For this review, take the finished solid that the model builds, in its own axes (mm). Round coordinates to 2 decimals unless told otherwise and drop trailing zeros. Write each loop counter-clockwise with the first axis right and the second up, starting at its lowest first coordinate (ties: lowest second). Pieces come first, ordered by that corner, then holes. Notation, with made-up numbers: (2, -25) -> (30, -25) arc R21 cw to (30, -6) -> close; hole circle Ø5 at (22, 34). An arc over 180 degrees is marked (long way). Answer in a Markdown table with one row per item. Add a question column.
```python
from build123d import *

# Parameters (mm, degrees)
SKETCH_1_W          = 17
SKETCH_1_H          = 14
SKETCH_1_R          = 1.1
EXTRUDE_1_DEPTH     = 3
EXTRUDE_3_DEPTH     = 3
SKETCH_3_R          = 1
CUT_EXTRUDE_1_DEPTH = 27.518861212
SKETCH_4_W          = 10
SKETCH_4_H          = 7
SKETCH_4_W_2        = 6
SKETCH_4_H_2        = 2
EXTRUDE_4_DEPTH     = 3
SKETCH_7_R          = 1
CUT_EXTRUDE_4_DEPTH = 27.518861212
FILLET_1_R          = 10
FILLET_2_R          = 2
CUT_EXTRUDE_5_DEPTH = 27.518861212


with BuildPart() as part:
    # 草图1 → 凸台-拉伸1 (new body)
    with BuildSketch(Plane(origin=(0, 0, 0), x_dir=(1, 0, 0), z_dir=(0, 1, 0))):
        Rectangle(SKETCH_1_W, SKETCH_1_H)
        with Locations(Location((-6, 4, 0), (0, 0, 270))):
            Circle(SKETCH_1_R, mode=Mode.SUBTRACT)
        with Locations(Location((6, 4, 0), (0, 0, 90))):
            Circle(SKETCH_1_R, mode=Mode.SUBTRACT)
        with Locations(Location((6, -4, 0), (0, 0, 270))):
            Circle(SKETCH_1_R, mode=Mode.SUBTRACT)
        with Locations(Location((-6, -4, 0), (0, 0, 90))):
            Circle(SKETCH_1_R, mode=Mode.SUBTRACT)
    extrude(amount=EXTRUDE_1_DEPTH)

    # 草图2 → 凸台-拉伸3 (add)
    with BuildSketch(Plane(origin=(0, 3, 0), x_dir=(1, 0, 0), z_dir=(0, 1, 0))):
        Polygon((5.5, 22), (5.5, 7), (8.5, 7), (8.5, -7), (14.5, 4), (14.5, 22), align=None)
    extrude(amount=-EXTRUDE_3_DEPTH)

    # 草图3 → 切除-拉伸1 (cut, through all)
    with BuildSketch(Plane(origin=(0, 3, 0), x_dir=(1, 0, 0), z_dir=(0, 1, 0))):
        with Locations(Location((8, 19, 0), (0, 0, 270))):
            Circle(SKETCH_3_R)
        with Locations(Location((8, 12, 0), (0, 0, 270))):
            Circle(SKETCH_3_R)
    extrude(amount=-CUT_EXTRUDE_1_DEPTH, mode=Mode.SUBTRACT)

    # 草图4 → 凸台-拉伸4 (add)
    with BuildSketch(Plane(origin=(0, 3, 0), x_dir=(1, 0, 0), z_dir=(0, 1, 0))):
        with Locations((0, -10.5)):
            Rectangle(SKETCH_4_W, SKETCH_4_H)
        with Locations((0, -11)):
            Rectangle(SKETCH_4_W_2, SKETCH_4_H_2, mode=Mode.SUBTRACT)
    extrude(amount=-EXTRUDE_4_DEPTH)

    # 草图7 → 切除-拉伸4 (cut, through all)
    with BuildSketch(Plane(origin=(0, 3, 0), x_dir=(1, 0, 0), z_dir=(0, 1, 0))):
        with Locations((5.707106781, -7.707106781)):
            Circle(SKETCH_7_R)
        with Locations((-5.707106781, -7.707106781)):
            Circle(SKETCH_7_R)
    extrude(amount=-CUT_EXTRUDE_4_DEPTH, mode=Mode.SUBTRACT)

    # 圆角1
    fillet_1_edges = [part.edges().sort_by_distance(p)[0] for p in [
        (14.5, 1.5, -4),
    ]]
    fillet(fillet_1_edges, radius=FILLET_1_R)

    # 圆角2
    fillet_2_edges = [part.edges().sort_by_distance(p)[0] for p in [
        (14.5, 1.5, -22),
        (5.5, 1.5, -22),
        (5.5, 1.5, -7),
        (8.5, 1.5, 7),
        (-8.5, 1.5, -7),
    ]]
    fillet(fillet_2_edges, radius=FILLET_2_R)

    # 草图8 → 切除-拉伸5 (cut, through all)
    with BuildSketch(Plane(origin=(0, 3, 0), x_dir=(1, 0, 0), z_dir=(0, 1, 0))):
        with BuildLine():
            ThreePointArc((-1.336748061, -11), (-2.292893219, -9.707106781), (-3.249038376, -11))
            ThreePointArc((-3.249038376, -11), (-2.292893219, -12.292893219), (-1.336748061, -11))
        make_face()
        with BuildLine():
            ThreePointArc((1.336748061, -11), (2.292893219, -12.292893219), (3.249038376, -11))
            ThreePointArc((3.249038376, -11), (2.292893219, -9.707106781), (1.336748061, -11))
        make_face()
    extrude(amount=-CUT_EXTRUDE_5_DEPTH, mode=Mode.SUBTRACT)


solid = part.part
```
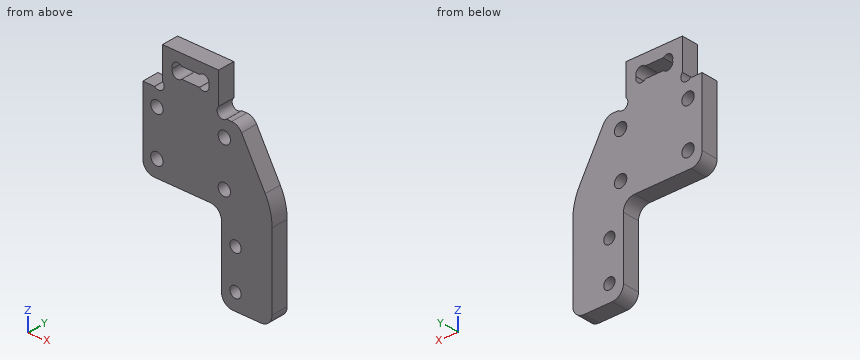
1. We need section C-C (x = -6). Write out the cut boundary in (y, z), plus the area to 3 significant figures.
2. We need section A-A (z = -12). Write out the cut boundary in (x, y).
3. We need section D-D (y = 0.75). Count the separate pieces of the cut face and the enclosed holes in it, plus the area to 3 significant figures.
4. Clearance check with flat-ended pins moving along their axes: pin 1 Ø1.5 at (y, z) = (2, -14.5) entering from -X; pin 2 Ø1.7 at (x, y) = (-7, 1.5) entering from +Z. State where each tip first meets the part, or that it passes through.
5. We need section B-B (x = 0.25). Write out the cut boundary in (y, z).
6. For L1, parallel to Z at x = -0.5, y = 2; L2, parallel to Z at x = 7.75, y = 2.25; L3, parallel to X at y = 0.85, z = -12, list the stretches that pass through material, from the lowest coordinate up. Write a range as [from, to].
Response:
| question | item | result |
|---|---|---|
| 1 | outline | (0, -7) -> (3, -7) -> (3, -5.1) -> (0, -5.1) -> close; (0, -2.9) -> (3, -2.9) -> (3, 2.9) -> (0, 2.9) -> close; (0, 5.1) -> (3, 5.1) -> (3, 6.75) -> (0, 6.75) -> close |
| 1 | area | 28.1 mm2 |
| 2 | outline | (5.5, 0) -> (7, 0) -> (7, 3) -> (5.5, 3) -> close; (9, 0) -> (14.5, 0) -> (14.5, 3) -> (9, 3) -> close |
| 3 | separate pieces | 1 |
| 3 | enclosed holes | 7 |
| 3 | area | 455 mm2 |
| 4 | pin 1 | x = 5.5 |
| 4 | pin 2 | z = 7 |
| 5 | outline | (0, -7) -> (3, -7) -> (3, 10) -> (0, 10) -> close; (0, 12) -> (3, 12) -> (3, 14) -> (0, 14) -> close |
| 6 | L1 | [-7, 10], [12, 14] |
| 6 | L2 | [-22, -19.97], [-18.03, -12.97], [-11.03, 6.95] |
| 6 | L3 | [5.5, 7], [9, 14.5] |
